Here's how the part is built. I have some questions about the finished solid (model axes, mm). Give positions to 0.01 mm unless a question says otherwise; leave off trailing zeros. Loops run counter-clockwise (first coordinate to the right, second up) from the corner with the lowest first, then second, coordinate; pieces in that order, holes last. Notation, with made-up numbers: (-35.75, 84) -> (12.25, 84) arc R26 cw to (12.25, 106) -> close; hole circle Ø1 at (70.5, -3). An arc over 180 degrees is marked (long way). Answer in a Markdown table with one row per item. Add a question column.
Item 1: For P1, Ø3, axis at x = 8.5, y = 94.5, coming from the -Z side, with a flat end and sliding along its axis, tell me the tip position at first contact or that it passes through.
Item 2: If I drill on line 1 (X direction, y = 94, z = 41); line 2 (Y direction, x = 4.5, z = 60); line 3 (X direction, y = 91.5, z = 81), over which ranges is the centre line in solid material (lowest first)?
Item 3: If we section it at A-A (z = 103): Write out the boundary of the cut face in (x, y).
Item 4: If we section it at C-C (x = 7): Write out the boundary of the cut face in (y, z), then the cut area to 3 significant figures.
Item 5: If we section it at B-B (y = 95.5): Write out the boundary of the cut face in (x, z), then the cut area to 3 significant figures.
```python
from build123d import *

# Parameters (mm, degrees)
EXTRUDE_1_DEPTH = 180


with BuildPart() as part:
    # 草图1 → 拉伸1 (new body)
    with BuildSketch(Plane.XY):
        with BuildLine():
            Line((11.786098163, 93.447548514), (11.185365906, 91.59914157))
            ThreePointArc((11.185365906, 91.59914157), (10.555305835, 91.278167571), (10.234331837, 91.908227642))
            Line((10.234331837, 91.908227642), (10.817155535, 93.701531326))
            ThreePointArc((10.817155535, 93.701531326), (10.82905345, 93.765700722), (10.823937692, 93.830763005))
            Line((10.823937692, 93.830763005), (10.12292529, 97.129945359))
            ThreePointArc((10.12292529, 97.129945359), (10.053162473, 97.243801851), (9.92729275, 97.28837723))
            Line((9.92729275, 97.28837723), (2.076289972, 97.28837723))
            ThreePointArc((2.076289972, 97.28837723), (1.94773245, 97.241586118), (1.879328421, 97.123106865))
            Line((1.879328421, 97.123106865), (1.291080466, 93.786986931))
            ThreePointArc((1.291080466, 93.786986931), (1.28823373, 93.721785951), (1.302359249, 93.658069851))
            Line((1.302359249, 93.658069851), (1.947284603, 91.886152004))
            ThreePointArc((1.947284603, 91.886152004), (1.648448364, 91.245295622), (1.007591982, 91.544131861))
            Line((1.007591982, 91.544131861), (0.339755623, 93.378997177))
            ThreePointArc((0.339755623, 93.378997177), (0.283253546, 93.633861578), (0.294640491, 93.894665498))
            Line((0.294640491, 93.894665498), (0.893043434, 97.28837723))
            Line((0.893043434, 97.28837723), (0.200002689, 97.28837723))
            ThreePointArc((0.200002689, 97.28837723), (0.058581333, 97.346955874), (2.689e-06, 97.48837723))
            Line((2.689e-06, 97.48837723), (2.689e-06, 97.98837723))
            ThreePointArc((2.689e-06, 97.98837723), (0.087870655, 98.200509264), (0.300002689, 98.28837723))
            Line((0.300002689, 98.28837723), (11.700002689, 98.28837723))
            ThreePointArc((11.700002689, 98.28837723), (11.912134724, 98.200509264), (12.000002689, 97.98837723))
            Line((12.000002689, 97.98837723), (12.000002689, 97.48837723))
            ThreePointArc((12.000002689, 97.48837723), (11.941424046, 97.346955874), (11.800002689, 97.28837723))
            Line((11.800002689, 97.28837723), (11.106961944, 97.28837723))
            Line((11.106961944, 97.28837723), (11.813226794, 93.96447523))
            ThreePointArc((11.813226794, 93.96447523), (11.833689825, 93.704226096), (11.786098163, 93.447548514))
        make_face()
    extrude(amount=EXTRUDE_1_DEPTH)


solid = part.part
```
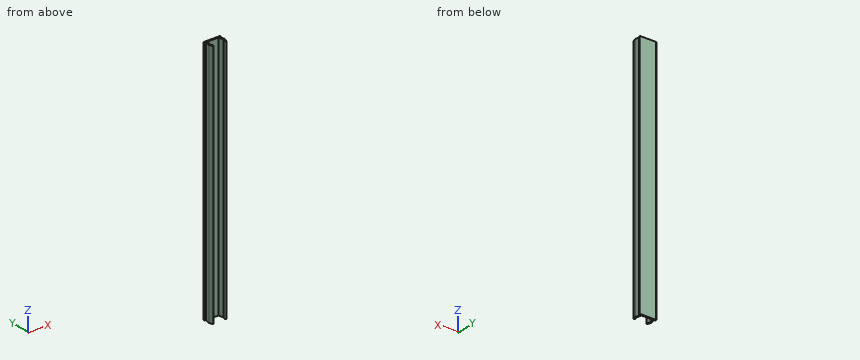
Recorded:
| question | item | result |
|---|---|---|
| 1 | P1 | passes through |
| 2 | line 1 | x = 0.31 to 1.33, 10.79 to 11.81 |
| 2 | line 2 | y = 97.29 to 98.29 |
| 2 | line 3 | x = 1.03 to 1.93, 10.28 to 11.14 |
| 3 | outline | (0, 97.49) arc R0.2 ccw to (0.2, 97.29) -> (0.89, 97.29) -> (0.29, 93.89) arc R1 ccw to (0.34, 93.38) -> (1.01, 91.54) arc R0.5 ccw to (1.95, 91.89) -> (1.3, 93.66) arc R0.25 cw to (1.29, 93.79) -> (1.88, 97.12) arc R0.2 cw to (2.08, 97.29) -> (9.93, 97.29) arc R0.2 cw to (10.12, 97.13) -> (10.82, 93.83) arc R0.25 cw to (10.82, 93.7) -> (10.23, 91.91) arc R0.5 ccw to (11.19, 91.6) -> (11.79, 93.45) arc R1 ccw to (11.81, 93.96) -> (11.11, 97.29) -> (11.8, 97.29) arc R0.2 ccw to (12, 97.49) -> (12, 97.99) arc R0.3 ccw to (11.7, 98.29) -> (0.3, 98.29) arc R0.3 ccw to (0, 97.99) -> close |
| 4 | outline | (97.29, 0) -> (98.29, 0) -> (98.29, 180) -> (97.29, 180) -> close |
| 4 | area | 180 mm^2 |
| 5 | outline | (0.58, 0) -> (1.59, 0) -> (1.59, 180) -> (0.58, 180) -> close; (10.47, 0) -> (11.49, 0) -> (11.49, 180) -> (10.47, 180) -> close |
| 5 | area | 366 mm^2 |
